from build123d import *

# Parameters (mm, degrees)
SKETCH1_W           = 60
SKETCH1_H           = 7
BOSS_EXTRUDE1_DEPTH = 10
SKETCH2_R           = 1.5
CUT_EXTRUDE1_DEPTH  = 5
FILLET1_R           = 4


with BuildPart() as part:
    # Sketch1 → Boss-Extrude1 (new body)
    with BuildSketch(Plane(origin=(0, 0, 0), x_dir=(1, 0, 0), z_dir=(0, 1, 0))):
        Rectangle(SKETCH1_W, SKETCH1_H)
    extrude(amount=BOSS_EXTRUDE1_DEPTH)

    # Sketch2 → Cut-Extrude1 (cut)
    with BuildSketch(Plane(origin=(0, 10, 0), x_dir=(1, 0, 0), z_dir=(0, 1, 0))):
        with Locations(Location((0, 0, 0), (0, 0, 270))):
            Circle(SKETCH2_R)
        with Locations(Location((20, 0, 0), (0, 0, 270))):
            Circle(SKETCH2_R)
        with Locations(Location((-20, 0, 0), (0, 0, 270))):
            Circle(SKETCH2_R)
    extrude(amount=-CUT_EXTRUDE1_DEPTH, mode=Mode.SUBTRACT)

    # Fillet1
    fillet1_edges = [part.edges().sort_by_distance(p)[0] for p in [
        (-30, 0, 0),
        (30, 0, 0),
    ]]
    fillet(fillet1_edges, radius=FILLET1_R)


solid = part.part
The listing builds one solid part. Answer for the finished solid, in the listing's coordinates (mm). A direction names the side the tool comes from. Coordinates: 2 decimals unless noted, no trailing zeros. Write each loop counter-clockwise with the first axis right and the second up, starting at its lowest first coordinate (ties: lowest second). Pieces come first, ordered by that corner, then holes. Notation, with made-up numbers: M -27,-40 L 29,-40 A36 cw 29,-3 Z; hole C -17,-27 d6. An arc over 180 degrees is marked long. Use one line per item in the form item = value.
Item 1: Given P1, Ø2.5, axis at x = 20, z = 0, coming from the +Y side; P2, Ø3.5, axis at x = 20, z = -0.5, coming from the +Y side, each flat-ended and moving along its own axis, determine where each tip first touches the part or whether it passes through.
Model answer:
P1 = 5
P2 = 10
Item 2: The mould has two halves that part along Z. Classify faces 3 (the face through (28.797, 1.141, -0.049)), 4 (the face through (-18.735, 7.535, 0.806)), 5 (the face through (0, 5, -3.5)): released by +Z, released by -Z, zero draft, split by the parting line, or undercut.
Model answer:
face_3 = zero draft
face_4 = undercut
face_5 = released by -Z
Item 3: Find section A-A, the plane z = 0. Give the vertices of the cut face in (x, y).
Model answer:
outline = M -30,4 A4 ccw -26,0 L 26,0 A4 ccw 30,4 L 30,10 L 21.5,10 L 21.5,5 L 18.5,5 L 18.5,10 L 1.5,10 L 1.5,5 L -1.5,5 L -1.5,10 L -18.5,10 L -18.5,5 L -21.5,5 L -21.5,10 L -30,10 Z
Item 4: Find section B-B, the plane x = 20. Give the vertices of the cut face in (y, z).
Model answer:
outline = M 0,-3.5 L 10,-3.5 L 10,-1.5 L 5,-1.5 L 5,1.5 L 10,1.5 L 10,3.5 L 0,3.5 Z
Item 5: Find the intervals of material crossed by probe 1 along X at (y, z) = (8.65, 0); probe 2 along X at (y, z) = (1.5, 3); probe 3 along X at (y, z) = (0.75, -2.5), in increasing order.
Model answer:
probe_1 = -30 to -21.5, -18.5 to -1.5, 1.5 to 18.5, 21.5 to 30
probe_2 = -29.12 to 29.12
probe_3 = -28.33 to 28.33
Item 6: For faces 1 (the face through (0, 0, 0)), 2 (the face through (0.45, 7.54, 1.43)), determine the directions among +Z, -Z, +X, -X, +Y, -Y from which every point of the face is accessible in a straight line to the end or side of a thin tool.
Model answer:
face_1 = +Z, -Z, +X, -X, -Y
face_2 = +Y
